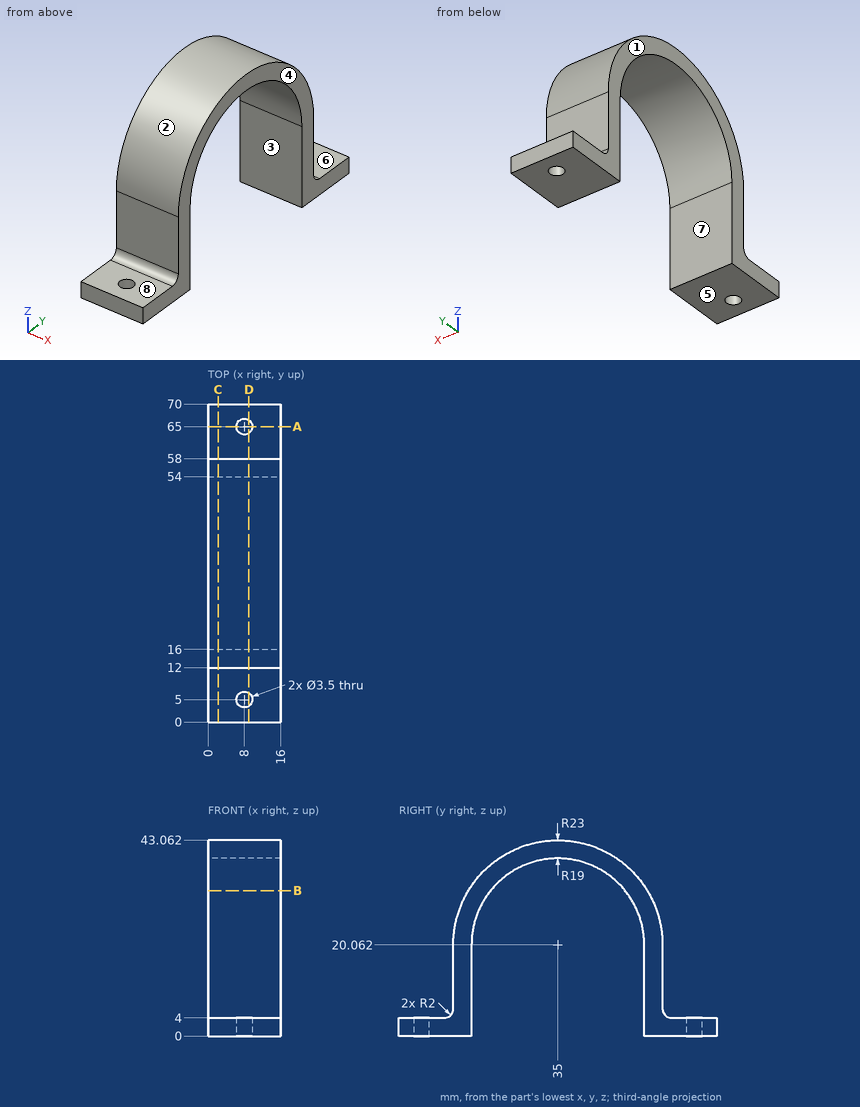
Check sheet for the drawn part. Datum: minimum x, y, z corner. Units: mm. A direction names the side the tool comes from. Round coordinates to 2 decimals unless told otherwise and drop trailing zeros. Loops run counter-clockwise (first coordinate to the right, second up) from the corner with the lowest first, then second, coordinate; pieces in that order, holes last.
Item 1: Cross-section at D-D on x = 9. Record the boundary of the cut face in (y, z), then the cut area to 3 significant figures.
Item 2: Cross-section at B-B on z = 32. Record the boundary of the cut face in (x, y), then the cut area to 3 significant figures.
Item 3: Cross-section at A-A on y = 65. Record the boundary of the cut face in (x, z), then the cut area to 3 significant figures.
Item 4: Mould release check, pull along Y, two halves, no side actions. Record for the marked faces 1, 2 and 3: pulls with the +Y half, pulls with the -Y half, needs draft (parallel to the pull), parting line crosses it, or undercut.
Item 5: Thickness scan on line 1 (Y direction, x = 9.75, z = 10); line 2 (X direction, y = 5, z = 2.15); line 3 (Y direction, x = 10.5, z = 2). Record the ranges inside material, lowest first.
Item 6: Access from +Z, -Z, +X, -X, +Y, -Y to the whole of each face (thin tool, end or side, straight path). Record for the marked faces 4, 5, 6, 7 and 8.
Item 7: Gauge pin test, flat ends, axial feed: pin 1 (2 mm diameter, centred on x = 8, y = 65, fed in from -Z); pin 2 (3 mm diameter, centred on x = 11, y = 51.5, fed in from +Z); pin 3 (2 mm diameter, centred on x = 5.5, y = 29, fed in from +Z); pin 4 (8 mm diameter, centred on x = 2, y = 26, fed in from -Z). Record the tip position at first contact, or that the pin passes through.
Item 8: Cross-section at C-C on x = 2.25. Record the boundary of the cut face in (y, z).
Answer sheet:
1. outline: (0, 0) - (3.56, 0) - (3.56, 4) - (0, 4) - close; (6.44, 0) - (16, 0) - (16, 20.06) arc R19 cw to (54, 20.06) - (54, 0) - (63.56, 0) - (63.56, 4) - (60, 4) arc R2 cw to (58, 6) - (58, 20.06) arc R23 ccw to (12, 20.06) - (12, 6) arc R2 cw to (10, 4) - (6.44, 4) - close; (66.44, 0) - (70, 0) - (70, 4) - (66.44, 4) - close
1. area: 499 mm2
2. outline: (0, 15.34) - (16, 15.34) - (16, 20.22) - (0, 20.22) - close; (0, 49.78) - (16, 49.78) - (16, 54.66) - (0, 54.66) - close
2. area: 156 mm2
3. outline: (0, 0) - (6.25, 0) - (6.25, 4) - (0, 4) - close; (9.75, 0) - (16, 0) - (16, 4) - (9.75, 4) - close
3. area: 50.0 mm2
4. face 1: needs draft
4. face 2: parting line crosses it
4. face 3: undercut
5. line 1: y = 12 to 16, 54 to 58
5. line 2: x = 0 to 6.25, 9.75 to 16
5. line 3: y = 0 to 16, 54 to 70
6. face 4: +Z, -Z, +X, +Y, -Y
6. face 5: -Z, +X, -X, +Y, -Y
6. face 6: +Z, +X, -X, +Y
6. face 7: -Z, +X, -X
6. face 8: +Z, +X, -X, -Y
7. pin 1: passes through
7. pin 2: stops at z = 37.5
7. pin 3: stops at z = 42.51
7. pin 4: stops at z = 33.92
8. outline: (0, 0) - (16, 0) - (16, 20.06) arc R19 cw to (54, 20.06) - (54, 0) - (70, 0) - (70, 4) - (60, 4) arc R2 cw to (58, 6) - (58, 20.06) arc R23 ccw to (12, 20.06) - (12, 6) arc R2 cw to (10, 4) - (0, 4) - close
